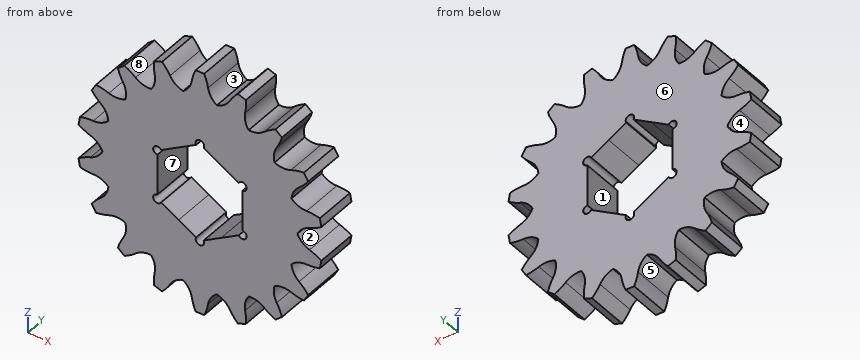
from build123d import *

# Parameters (mm, degrees)
BOSS_EXTRUDE1_DEPTH = 5
CIRPATTERN2_COUNT   = 18
BOSS_EXTRUDE3_DEPTH = 5


with BuildPart() as part:
    # Sketch1 → Boss-Extrude1 (new body)
    with BuildSketch(Plane(origin=(0, 0, 0), x_dir=(1, 0, 0), z_dir=(0, 1, 0))):
        with BuildLine():
            Line((0.5, 14.415439282), (-0.5, 14.415439282))
            ThreePointArc((-0.5, 14.415439282), (-0.952778657, 12.949235725), (-1, 11.415439282))
            Line((-1, 11.415439282), (1, 11.415439282))
            ThreePointArc((1, 11.415439282), (0.952778657, 12.949235725), (0.5, 14.415439282))
        make_face()
        with BuildLine():
            Line((0, 12.915439282), (0.9583076, 12.915439282))
            ThreePointArc((0.9583076, 12.915439282), (1.309947673, 11.991364327), (2, 11.283273195))
            Line((2, 11.283273195), (-2, 11.283273195))
            ThreePointArc((-2, 11.283273195), (-1.309947673, 11.991364327), (-0.9583076, 12.915439282))
            Line((-0.9583076, 12.915439282), (0, 12.915439282))
        make_face()
    boss_extrude1 = extrude(amount=BOSS_EXTRUDE1_DEPTH)

    # CirPattern2: Boss-Extrude1 ×18 about axis
    cirpattern2_axis = Axis((0, 0, 0), (0, 1, 0))
    for i in range(1, CIRPATTERN2_COUNT):
        add(boss_extrude1.rotate(cirpattern2_axis, i * 360 / CIRPATTERN2_COUNT))

    # Sketch1<5> → Boss-Extrude3 (add)
    with BuildSketch(Plane(origin=(0, 0, 0), x_dir=(1, 0, 0), z_dir=(0, 1, 0))):
        with BuildLine():
            ThreePointArc((11.459155903, 0), (8.781530784, 7.361859215), (2, 11.283273195))
            Line((2, 11.283273195), (-2, 11.283273195))
            ThreePointArc((-2, 11.283273195), (-7.361859215, -8.781530784), (11.459155903, 0))
        make_face()
        with BuildLine():
            Line((-0.433012702, -5.523502692), (-2.500000064, -4.330126982))
            Line((-2.500000064, -4.330126982), (-4.566987298, -3.136751346))
            ThreePointArc((-4.566987298, -3.136751346), (-5.433012702, -3.136751346), (-5, -2.386751346))
            Line((-5, -2.386751346), (-5, -2e-09))
            Line((-5, -2e-09), (-5, 2.386751346))
            ThreePointArc((-5, 2.386751346), (-5.433012702, 3.136751346), (-4.566987298, 3.136751346))
            Line((-4.566987298, 3.136751346), (-2.499999953, 4.330127046))
            Line((-2.499999953, 4.330127046), (-0.433012702, 5.523502692))
            ThreePointArc((-0.433012702, 5.523502692), (-0.129409523, 6.256465605), (0.5, 5.773502692))
            ThreePointArc((0.5, 5.773502692), (0.482962913, 5.644093169), (0.433012702, 5.523502692))
            Line((0.433012702, 5.523502692), (2.500000011, 4.330127013))
            Line((2.500000011, 4.330127013), (4.566987298, 3.136751346))
            ThreePointArc((4.566987298, 3.136751346), (5.129409523, 3.369714259), (5.5, 2.886751346))
            ThreePointArc((5.5, 2.886751346), (5.353553391, 2.533197955), (5, 2.386751346))
            Line((5, 2.386751346), (5, 0))
            Line((5, 0), (5, -2.386751346))
            ThreePointArc((5, -2.386751346), (5.353553391, -2.533197955), (5.5, -2.886751346))
            ThreePointArc((5.5, -2.886751346), (5.129409523, -3.369714259), (4.566987298, -3.136751346))
            Line((4.566987298, -3.136751346), (2.499999978, -4.330127032))
            Line((2.499999978, -4.330127032), (0.433012702, -5.523502692))
            ThreePointArc((0.433012702, -5.523502692), (0.482962913, -5.644093169), (0.5, -5.773502692))
            ThreePointArc((0.5, -5.773502692), (-0.129409523, -6.256465605), (-0.433012702, -5.523502692))
        make_face(mode=Mode.SUBTRACT)
    extrude(amount=BOSS_EXTRUDE3_DEPTH)


solid = part.part
Build history of the part. All positions in model axes, mm. Face numbers are marked on the shaded views. A direction names the side the tool comes from. Round coordinates to 2 decimals unless told otherwise and drop trailing zeros. Write each loop counter-clockwise with the first axis right and the second up, starting at its lowest first coordinate (ties: lowest second). Pieces come first, ordered by that corner, then holes. Notation, with made-up numbers: (68.5, 79.25) -> (78.5, 79.25) arc R21 ccw to (78.5, 85.25) -> close; hole circle Ø8 at (32, -34). An arc over 180 degrees is marked (long way). Write item = value, one per line.
(1) Flat gauge pins, fed straight in: pin 1 (0.9 mm diameter, centred on x = 0, z = 5.77, fed in from +Y); pin 2 (1.5 mm diameter, centred on x = 6, y = 1, fed in from -Z). Where does each tip first touch, or does it go through?
Answer:
pin_1 = through
pin_2 = -13.43
(2) Band-saw the part on C-C (x = 6.25). Give the cut face in (y, z).
Answer:
outline = (0, -9.93) -> (5, -9.93) -> (5, 9.93) -> (0, 9.93) -> close
(3) Two-plate mould, pull along Z, no slides. Class the marked faces 6, 7 and 8: pulls with the +Z half, pulls with the -Z half, needs draft (parallel to the pull), parting line crosses it, or undercut.
Answer:
face_6 = needs draft
face_7 = undercut
face_8 = pulls with the +Z half
(4) Band-saw the part on B-B (z = -8). Give the cut face in (x, y), then the cut area to 3 significant figures.
Answer:
outline = (-8.69, 0) -> (8.69, 0) -> (8.69, 5) -> (-8.69, 5) -> close
area = 86.9 mm2
(5) Tool access for the marked faces 1, 2, 3, 4 and 5: list every direction of +Z, -Z, +X, -X, +Y, -Y with a clear straight run to the whole face (end or side of a thin tool).
Answer:
face_1 = +Y, -Y
face_2 = +X, +Y, -Y
face_3 = +Z, +Y, -Y
face_4 = -X, +Y, -Y
face_5 = -Z, +Y, -Y
(6) Band-saw the part on A-A (x = 0). Give the cut face in (y, z), then the cut area to 3 significant figures.
Answer:
outline = (0, -14.42) -> (5, -14.42) -> (5, -6.27) -> (0, -6.27) -> close; (0, 6.27) -> (5, 6.27) -> (5, 14.42) -> (0, 14.42) -> close
area = 81.4 mm2
(7) Probe L1, parallel to Z at x = 0, y = 3.85; L2, parallel to Z at x = 9, y = 3.2; L3, parallel to X at y = 4.4, z = -10.25. List the from-to ranges inside material, lowest first.
Answer:
L1 = -14.42 to -6.27, 6.27 to 14.42
L2 = -11.27 to -9.22, -7.28 to 7.28, 9.22 to 11.27
L3 = -9.5 to -7.21, -5.54 to 5.54, 7.21 to 9.5
